Geometry check sheet. Reference: the model listing, model coordinates, mm. Face numbers are marked on the shaded views. Give positions to 0.01 mm unless a question says otherwise; leave off trailing zeros. Order: outer loops, then holes, each group sorted by start corner. A loop starts at its lowest first (then second) coordinate and runs counter-clockwise, first axis right, second up.
Solid Edge part; units mm, degrees
sketch "Sketch1" plane through (10.8674, 10.8674, 0) normal (0, 0, 1) x (1, 0, 0)
  line L0 (-14.9088, -10.8674) -> (-12.8881, -7.3674)
  line L1 (-12.8881, -7.3674) -> (-8.8467, -7.3674)
  line L2 (-8.8467, -7.3674) -> (-6.8259, -10.8674)
  line L3 (-6.8259, -10.8674) -> (-8.8467, -14.3674)
  line L4 (-8.8467, -14.3674) -> (-12.8881, -14.3674)
  line L5 (-12.8881, -14.3674) -> (-14.9088, -10.8674)
extrude "Protrusion1" add sketch "Sketch1" along normal mid plane 3.2
sketch "Sketch2" plane through (0, 8.3963, 8.3963) normal (1, 0, 0) x (0, 1, 0)
  line L0 (-11.8963, -6.7963) -> (-14.6675, -8.3963)
  line L1 (-14.6675, -8.3963) -> (-11.8963, -9.9963)
revolve "RevolvedCutout1" cut sketch "Sketch2" angle 360 about axis through (0, 0, 1.6) along (0, 0, -1) material side at (0, -4.9106, 0.8433)
hole "Hål_M6" at (0, 0, 1.6) direction (0, 0, -1) diameter 4.917 end up to next
properties material "Iron"
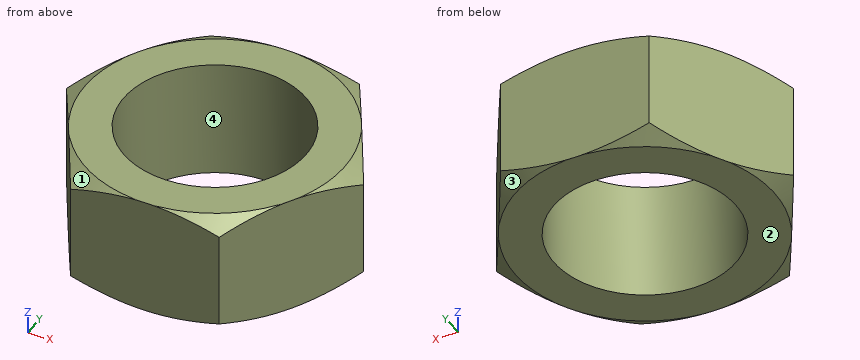
Item 1: Sectioned sample at A-A (z = 0.55). Enter the section's corners in (x, y).
Reported:
outline: (-4.04, 0) - (-2.02, -3.5) - (2.02, -3.5) - (4.04, 0) - (2.02, 3.5) - (-2.02, 3.5) - close; hole circle Ø4.92 at (0, 0)
Item 2: Scan lines: L1, parallel to Y at x = 0, z = -0.7; L2, parallel to Y at x = 0.25, z = -1.3; L3, parallel to X at y = 0.75, z = -0.4. Record each from-to range of solid material in increasing order.
Reported:
L1: y = -3.5 to -2.46, 2.46 to 3.5
L2: y = -3.5 to -2.45, 2.45 to 3.5
L3: x = -3.61 to -2.34, 2.34 to 3.61
Item 3: Draft check along X on the marked faces 1, 2, 3 and 4. Enter one of: released by +X, released by -X, zero draft, split by the parting line, or undercut.
Reported:
face 1: released by -X
face 2: zero draft
face 3: released by +X
face 4: undercut
